For this review, use the dimensioned drawing (mm, ordinates from the lowest corner) and the shaded views. Round coordinates to 2 decimals unless told otherwise and drop trailing zeros. Loops run counter-clockwise (first coordinate to the right, second up) from the corner with the lowest first, then second, coordinate; pieces in that order, holes last. Notation, with made-up numbers: (-31, -19) -> (-11, -19) arc R5 ccw to (-11, -11) -> close; hole circle Ø7 at (61.5, 4). An arc over 180 degrees is marked (long way). Answer as CSV lines item,"result". Start each with the question number.
(1) To check wall thickness, follow line 1 (Z direction, x = 25.4, y = 0.9) (3 decimals); line 2 (Y direction, x = 22, z = 37.5) (3 decimals). State the ranges of each line that lie inside material, in increasing order. Write a range as from..to.
(2) For P1, Ø9.5, axis at x = 17.5, z = 26, coming from the -Y side (3 decimals), flat-tipped, find the tip position at first contact; note if it passes through.
(3) Take a section at A-A, the plane x = 25.4. Write out the cut boundary in (y, z) (3 decimals), and give its area (3 significant figures).
(4) Draft analysis for pull direction Z (two halves, no side actions). For the marked faces 1, 2 and 3, state which applies: +Z half, -Z half, draft (parallel to the pull), parting line (faces both ways), or undercut.
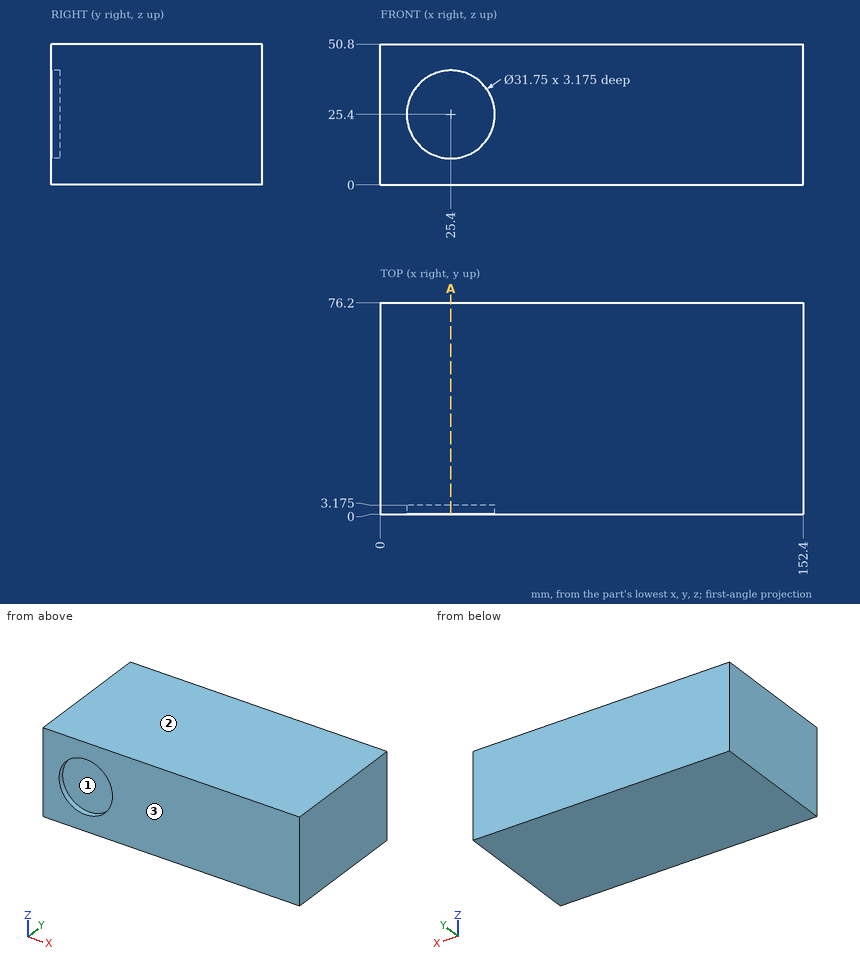
The answers:
1,line 1,"0..9.525, 41.275..50.8"
1,line 2,"3.175..76.2"
2,P1,"y = 3.175"
3,outline,"(0, 0) -> (76.2, 0) -> (76.2, 50.8) -> (0, 50.8) -> (0, 41.275) -> (3.175, 41.275) -> (3.175, 9.525) -> (0, 9.525) -> close"
3,area,"3,770 mm²"
4,face 1,"undercut"
4,face 2,"+Z half"
4,face 3,"draft"
